from build123d import *

# Parameters (mm, degrees)
SKETCH1_W           = 83
SKETCH1_H           = 83
BOSS_EXTRUDE1_DEPTH = 3
SKETCH2_W           = 13
SKETCH2_H           = 25
CUT_EXTRUDE1_DEPTH  = 3
CHAMFER1_SIZE       = 3.5
SKETCH3_W           = 15
SKETCH3_H           = 3
SKETCH3_W_2         = 3
SKETCH3_H_2         = 15
BOSS_EXTRUDE2_DEPTH = 3
SKETCH4_W           = 3
SKETCH4_H           = 612
BOSS_EXTRUDE3_DEPTH = 1
SKETCH5_W           = 175
SKETCH5_H           = 3
BOSS_EXTRUDE4_DEPTH = 1


with BuildPart() as part:
    # Sketch1 → Boss-Extrude1 (new body)
    with BuildSketch(Plane.XY):
        Rectangle(SKETCH1_W, SKETCH1_H)
    extrude(amount=BOSS_EXTRUDE1_DEPTH)

    # Sketch2 → Cut-Extrude1 (cut)
    with BuildSketch(Plane.XY.offset(3)):
        with Locations((0, 25.5)):
            Rectangle(SKETCH2_W, SKETCH2_H)
        with Locations((0, -25.5)):
            Rectangle(SKETCH2_W, SKETCH2_H)
    extrude(amount=-CUT_EXTRUDE1_DEPTH, mode=Mode.SUBTRACT)

    # Chamfer1
    chamfer1_edges = [part.edges().sort_by_distance(p)[0] for p in [
        (-41.5, 41.5, 1.5),
        (41.5, 41.5, 1.5),
        (41.5, -41.5, 1.5),
        (-41.5, -41.5, 1.5),
    ]]
    chamfer(chamfer1_edges, length=CHAMFER1_SIZE)

    # Sketch3 → Boss-Extrude2 (add)
    with BuildSketch(Plane.XY.offset(3)):
        with Locations((-26, -1)):
            Rectangle(SKETCH3_W, SKETCH3_H)
        with Locations((25, 22)):
            Rectangle(SKETCH3_W_2, SKETCH3_H_2)
    extrude(amount=BOSS_EXTRUDE2_DEPTH)

    # Sketch4 → Boss-Extrude3 (add)
    with BuildSketch(Plane.ZY.offset(-23.5)):
        with Locations((4.5, -276.5)):
            Rectangle(SKETCH4_W, SKETCH4_H)
    extrude(amount=BOSS_EXTRUDE3_DEPTH)

    # Sketch5 → Boss-Extrude4 (add)
    with BuildSketch(Plane.XZ.offset(2.5)):
        with Locations((-106, 4.5)):
            Rectangle(SKETCH5_W, SKETCH5_H)
    extrude(amount=BOSS_EXTRUDE4_DEPTH)


solid = part.part
Geometry: final body of the model. Coordinates: model frame, mm. Round coordinates to 2 decimals unless told otherwise and drop trailing zeros. Order: outer loops, then holes, each group sorted by start corner. A loop starts at its lowest first (then second) coordinate and runs counter-clockwise, first axis right, second up. Notation, with made-up numbers: (68, -23.75) -> (74, -23.75) arc R30 cw to (74, -0.75) -> close; hole circle Ø11 at (14.25, 0). An arc over 180 degrees is marked (long way). Put each result on its own line as item: value. Start each with the question number.
Q1. Line query: probe 1 along Y at (x, z) = (-3, 1); probe 2 along Y at (x, z) = (-112.5, 3.2); probe 3 along X at (y, z) = (-60.5, 4.65). Output: solid intervals per line, ascending.
Q2. Section A-A on z = 4.95. Return the cut outline in (x, y), and give its area (3 significant figures).
Q3. Section B-B on x = -126. Return the cut outline in (y, z).
Q4. First-contact query: pin 1 (2.5 mm diameter, centred on y = 21.5, z = 5, fed in from +X); pin 2 (1.5 mm diameter, centred on y = -29, z = 2, fed in from -X); pin 3 (2.5 mm diameter, centred on y = -283.5, z = 4, fed in from +X). Flat tips, straight axial feed; report the tip coordinate or a pass-through.
Q5. Section C-C on y = -268. Return the cut outline in (x, z), and give its area (3 significant figures).
Ans:
1. probe 1: y = -41.5 to -38, -13 to 13, 38 to 41.5
1. probe 2: y = -3.5 to -2.5
1. probe 3: x = 22.5 to 23.5
2. outline: (-193.5, -3.5) -> (-18.5, -3.5) -> (-18.5, 0.5) -> (-33.5, 0.5) -> (-33.5, -2.5) -> (-193.5, -2.5) -> close; (22.5, -582.5) -> (23.5, -582.5) -> (23.5, 14.5) -> (26.5, 14.5) -> (26.5, 29.5) -> (22.5, 29.5) -> close
2. area: 877 mm2
3. outline: (-3.5, 3) -> (-2.5, 3) -> (-2.5, 6) -> (-3.5, 6) -> close
4. pin 1: stops at x = 26.5
4. pin 2: stops at x = -41.5
4. pin 3: stops at x = 23.5
5. outline: (22.5, 3) -> (23.5, 3) -> (23.5, 6) -> (22.5, 6) -> close
5. area: 3.00 mm2
